The listing builds one solid part. Answer for the finished solid, in the listing's coordinates (mm). A direction names the side the tool comes from. Give positions to 0.01 mm unless a question says otherwise; leave off trailing zeros. Write each loop counter-clockwise with the first axis right and the second up, starting at its lowest first coordinate (ties: lowest second). Pieces come first, ordered by that corner, then holes. Notation, with made-up numbers: (45.25, -13.75) - (68.25, -13.75) arc R9 cw to (68.25, -4.75) - close; hole circle Ø6 at (77, 21). An arc over 180 degrees is marked (long way). One line per question, with ' | ' between items. Start each with the question number.
1. Find the intervals of material crossed by L1, parallel to Z at x = -33.75, y = -0.2; L2, parallel to Z at x = 0, y = -0.7 (3 decimals); L3, parallel to X at y = -1.55, z = 5, in increasing order. Write a range as from..to.
2. For faces 3 (the face through (31, 0, 1)), 4 (the face through (0.3, -1.5, 37.5)), determine the directions among +Z, -Z, +X, -X, +Y, -Y from which every point of the face is accessible in a straight line to the end or side of a thin tool.
3. Given P1, Ø1, axis at x = 22.5, z = -24.5, coming from the -Y side, flat-ended and moving along its own axis, determine where the tip first touches the part or whether it passes through.
4. The mould has two halves that part along Z. Classify faces 1 (the face through (-29.97, -0.51, 1.32)), 2 (the face through (0, -2, 38)): +Z half, -Z half, draft (parallel to the pull), parting line (faces both ways), or undercut.
5. A cutting plane is placed at A-A (y = -1.5). Determine the outline of the cut face in (x, z).
6. A cutting plane is placed at B-B (z = -8). Determine the outline of the cut face in (x, y), then the cut area to 3 significant figures.
7. A cutting plane is placed at C-C (x = 52). Determine the outline of the cut face in (y, z), then the cut area to 3 significant figures.
```python
from build123d import *

# Parameters (mm, degrees)
F0_W     = 145
F0_H     = 84
F1_DEPTH = 2
F3_DEPTH = 1
F4_R     = 30
F5_DEPTH = 25
F6_R     = 1
F7_DEPTH = 25
F8_R     = 1
F9_DEPTH = 25
F10_R    = 5


with BuildPart() as f1:
    # F0 (on Front) → F1 (new body)
    with BuildSketch(Plane.XZ):
        Rectangle(F0_W, F0_H)
    extrude(amount=F1_DEPTH)

    # F2 (on face) → F3 (cut)
    with BuildSketch(Plane.XZ.offset(2)):
        with BuildLine():
            ThreePointArc((18.7082869339, -32.5), (32.4639088837, -18.7708449461), (37.5, 0))
            ThreePointArc((37.5, 0), (32.4639088837, 18.7708449461), (18.7082869339, 32.5))
            Line((18.7082869339, 32.5), (-18.7082869339, 32.5))
            ThreePointArc((-18.7082869339, 32.5), (-37.5, 0), (-18.7082869339, -32.5))
            Line((-18.7082869339, -32.5), (18.7082869339, -32.5))
        make_face()
        with BuildLine():
            ThreePointArc((18.7082869339, 32.5), (32.4639088837, 18.7708449461), (37.5, 0))
            ThreePointArc((37.5, 0), (32.4639088837, -18.7708449461), (18.7082869339, -32.5))
            Line((18.7082869339, -32.5), (63.75, -32.5))
            Line((63.75, -32.5), (63.75, 32.5))
            Line((63.75, 32.5), (18.7082869339, 32.5))
        make_face()
        with BuildLine():
            Line((-18.7082869339, 32.5), (18.7082869339, 32.5))
            ThreePointArc((18.7082869339, 32.5), (0, 37.5), (-18.7082869339, 32.5))
        make_face()
        with BuildLine():
            ThreePointArc((-18.7082869339, -32.5), (0, -37.5), (18.7082869339, -32.5))
            Line((18.7082869339, -32.5), (-18.7082869339, -32.5))
        make_face()
        with BuildLine():
            ThreePointArc((-18.7082869339, -32.5), (-37.5, 0), (-18.7082869339, 32.5))
            Line((-18.7082869339, 32.5), (-63.75, 32.5))
            Line((-63.75, 32.5), (-63.75, -32.5))
            Line((-63.75, -32.5), (-18.7082869339, -32.5))
        make_face()
    extrude(amount=-F3_DEPTH, mode=Mode.SUBTRACT)

    # F4 (on face) → F5 (cut)
    with BuildSketch(Plane.XZ.offset(1)):
        Circle(F4_R)
    extrude(amount=-F5_DEPTH, mode=Mode.SUBTRACT)

    # F6 (on face) → F7 (cut)
    with BuildSketch(Plane.XZ.offset(1)):
        with Locations((-58.75, 27.5)):
            Circle(F6_R)
        with Locations((-58.75, -27.5)):
            Circle(F6_R)
        with Locations((58.75, -27.5)):
            Circle(F6_R)
        with Locations((58.75, 27.5)):
            Circle(F6_R)
        with Locations((-58.75, 0)):
            Circle(F6_R)
        with Locations((58.75, 0)):
            Circle(F6_R)
        with Locations((-33.75, 27.5)):
            Circle(F6_R)
        with Locations((33.75, 27.5)):
            Circle(F6_R)
        with Locations((33.75, -27.5)):
            Circle(F6_R)
        with Locations((-33.75, -27.5)):
            Circle(F6_R)
    extrude(amount=-F7_DEPTH, mode=Mode.SUBTRACT)

    # F8 (on face) → F9 (cut)
    with BuildSketch(Plane.XZ.offset(1)):
        with Locations((0, 33.875)):
            Circle(F8_R)
        with Locations((33.875, 0)):
            Circle(F8_R)
        with Locations((-33.875, 0)):
            Circle(F8_R)
        with Locations((0, -33.875)):
            Circle(F8_R)
    extrude(amount=-F9_DEPTH, mode=Mode.SUBTRACT)

    # F10
    f10_edges = [f1.edges().sort_by_distance(p)[0] for p in [
        (-63.75, -1.5, 32.5),
        (-63.75, -1.5, -32.5),
        (63.75, -1.5, 32.5),
        (63.75, -1.5, -32.5),
    ]]
    fillet(f10_edges, radius=F10_R)


solid = f1.part
```
Determined:
1) L1: -42..-28.5, -26.5..-0.99, 0.99..26.5, 28.5..42 | L2: -42..-34.875, -32.875..-30, 30..32.875, 34.875..42 | L3: -72.5..-63.75, 63.75..72.5
2) face 3: +Z, -Z, +X, -X, +Y | face 4: -Y
3) P1: y = -1
4) face 1: undercut | face 2: draft
5) outline: (-72.5, -42) - (72.5, -42) - (72.5, 42) - (-72.5, 42) - close; hole (-63.75, -27.5) arc R5 ccw to (-58.75, -32.5) - (-18.71, -32.5) arc R37.5 ccw to (18.71, -32.5) - (58.75, -32.5) arc R5 ccw to (63.75, -27.5) - (63.75, 27.5) arc R5 ccw to (58.75, 32.5) - (18.71, 32.5) arc R37.5 ccw to (-18.71, 32.5) - (-58.75, 32.5) arc R5 ccw to (-63.75, 27.5) - close
6) outline: (-72.5, -2) - (-63.75, -2) - (-63.75, -1) - (-28.91, -1) - (-28.91, 0) - (-72.5, 0) - close; (28.91, -1) - (63.75, -1) - (63.75, -2) - (72.5, -2) - (72.5, 0) - (28.91, 0) - close | area: 105 mm2
7) outline: (-2, -42) - (0, -42) - (0, 42) - (-2, 42) - (-2, 32.5) - (-1, 32.5) - (-1, -32.5) - (-2, -32.5) - close | area: 103 mm2
